The listing builds one solid part. Answer for the finished solid, in the listing's coordinates (mm). A direction names the side the tool comes from. Give positions to 0.01 mm unless a question says otherwise; leave off trailing zeros. Order: outer loops, then holes, each group sorted by start corner. A loop starts at its lowest first (then second) coordinate and runs counter-clockwise, first axis right, second up. Notation, with made-up numbers: (0, -23.75) - (20, -23.75) arc R19 ccw to (20, -2.75) - close; hole circle Ø10 at (-26.75, 35). An arc over 180 degrees is marked (long way). Answer as a JSON object with one key per item and string values. Group by question number.
Q1. The mould has two halves that part along X. Classify faces 1 (the face through (3.49, 2.05, -0.65)), 2 (the face through (0.13, 4.08, 0.08)), 3 (the face through (1, 0.8, 0)): released by +X, released by -X, zero draft, split by the parting line, or undercut.
Q2. Given pin 1 (1 mm diameter, centred on x = 0.5, z = -2, fed in from -Y); pin 2 (0.8 mm diameter, centred on y = 0.5, z = -2, fed in from -X); pin 3 (3 mm diameter, centred on y = 0.5, z = -3.5, fed in from +X); pin 4 (1.5 mm diameter, centred on x = 1, z = 3, fed in from -Y), each flat-ended and moving along its own axis, determine where each tip first touches the part or whether it passes through.
Q3. Consider line 1 (X direction, y = -0.75, z = -3); line 2 (X direction, y = -2.75, z = 2); line 3 (X direction, y = 0.5, z = -2.75). Determine where each line is inside the solid, lowest interval first.
Q4. A cutting plane is placed at B-B, the plane x = 3.5. Give the vertices of the cut face in (y, z).
Q5. For faces 4 (the face through (1, -0.8, 0)), 5 (the face through (8, -3, 0)), 6 (the face through (0, 2, 0)), determine the directions among +Z, -Z, +X, -X, +Y, -Y from which every point of the face is accessible in a straight line to the end or side of a thin tool.
Q6. A cutting plane is placed at A-A, the plane x = 1. Give the vertices of the cut face in (y, z).
Q7. A cutting plane is placed at C-C, the plane x = 7. Give the vertices of the cut face in (y, z), and give its area (3 significant figures).
from build123d import *

# Parameters (mm, degrees)
CHAMFER_1_SIZE           = 1
FILLET_1_R               = 0.6
CHAMFER_2_SIZE           = 0.8
SKETCH_2_W               = 1.2
SKETCH_2_H               = 1.6
CUT_EXTRUDE_1_DEPTH      = 5.75
CUT_EXTRUDE_1_DEPTH_BACK = 5.75


with BuildPart() as part:
    # Эскиз1 → Повернуть1 (revolve)
    with BuildSketch(Plane.XY):
        Polygon((0, 0), (0, 4.75), (1.8, 4.75), (1.8, 2.15), (4.8, 2.15), (5.65, 3), (10.3, 3), (10.3, 0), align=None)
    revolve(axis=Axis((0, 0, 0), (-1, 0, 0)))

    # Фаска1
    chamfer_1_edges = [part.edges().sort_by_distance(p)[0] for p in [
        (10.3, -3, 0),
    ]]
    chamfer(chamfer_1_edges, length=CHAMFER_1_SIZE)

    # Скругление1
    fillet_1_edges = [part.edges().sort_by_distance(p)[0] for p in [
        (4.8, -2.15, 0),
        (1.8, -2.15, 0),
    ]]
    fillet(fillet_1_edges, radius=FILLET_1_R)

    # Фаска2
    chamfer_2_edges = [part.edges().sort_by_distance(p)[0] for p in [
        (0, -4.75, 0),
    ]]
    chamfer(chamfer_2_edges, length=CHAMFER_2_SIZE)

    # Эскиз2 → Вырез-Вытянуть1 (cut, two sides)
    with BuildSketch(Plane.XY) as cut_extrude_1_sk:
        with Locations((0.6, 0)):
            Rectangle(SKETCH_2_W, SKETCH_2_H)
    extrude(amount=CUT_EXTRUDE_1_DEPTH, mode=Mode.SUBTRACT)
    extrude(cut_extrude_1_sk.sketch, amount=-CUT_EXTRUDE_1_DEPTH_BACK, mode=Mode.SUBTRACT)


solid = part.part
Reply:
{
 "1": {"face 1": "undercut", "face 2": "released by -X", "face 3": "zero draft"},
 "2": {"pin 1": "stops at y = -4.47", "pin 2": "stops at x = 0", "pin 3": "stops at x = 10.26", "pin 4": "stops at y = -4.18"},
 "3": {"line 1": "x = 1.2 to 1.8", "line 2": "x = 0 to 1.8", "line 3": "x = 1.2 to 1.8, 5.45 to 9.5"},
 "4": {"outline": "circle Ø4.3 at (0, 0)"},
 "5": {"face 4": "+Z, -Z, -X", "face 5": "+X", "face 6": "+Z, -Z, -X, +Y, -Y"},
 "6": {"outline": "(-0.8, -4.68) - (-0.8, 4.68) arc R4.75 ccw to start; (0.8, -4.68) arc R4.75 ccw to (0.8, 4.68) - close"},
 "7": {"outline": "circle Ø6 at (0, 0)", "area": "28.3 mm^2"}
}
